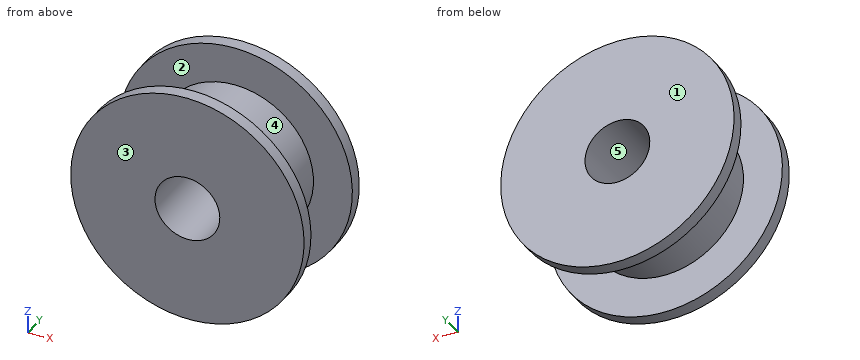
from build123d import *

# Parameters (mm, degrees)
SKETCH1_R           = 9
BOSS_EXTRUDE1_DEPTH = 8
SKETCH3_R           = 2.5
CUT_EXTRUDE1_DEPTH  = 16.033296378
SKETCH2_W           = 3
SKETCH2_H           = 6


with BuildPart() as part:
    # Sketch1 → Boss-Extrude1 (new body)
    with BuildSketch(Plane(origin=(0, 0, 0), x_dir=(1, 0, 0), z_dir=(0, 1, 0))):
        with Locations(Location((0, 0, 0), (0, 0, 270))):
            Circle(SKETCH1_R)
    extrude(amount=BOSS_EXTRUDE1_DEPTH)

    # Sketch3 → Cut-Extrude1 (cut, through all)
    with BuildSketch(Plane(origin=(0, 8, 0), x_dir=(1, 0, 0), z_dir=(0, 1, 0))):
        with Locations(Location((0, 0, 0), (0, 0, 270))):
            Circle(SKETCH3_R)
    extrude(amount=-CUT_EXTRUDE1_DEPTH, mode=Mode.SUBTRACT)

    # Sketch2 → Cut-Revolve1 (revolve, cut)
    with BuildSketch(Plane(origin=(0, 0, 0), x_dir=(0, 0, -1), z_dir=(1, 0, 0)), mode=Mode.PRIVATE) as cut_revolve1_sk:
        with Locations((-7.5, 4)):
            Rectangle(SKETCH2_W, SKETCH2_H)
    revolve(cut_revolve1_sk.sketch.rotate(Axis((0, 0, 0), (0, 1, 0)), 180), axis=Axis((0, 0, 0), (0, 1, 0)), mode=Mode.SUBTRACT)


solid = part.part
Verification items for the finished model (mm, model axes). Face numbers are marked on the shaded views. A direction names the side the tool comes from. Give positions to 0.01 mm unless a question says otherwise; leave off trailing zeros. Write each loop counter-clockwise with the first axis right and the second up, starting at its lowest first coordinate (ties: lowest second). Pieces come first, ordered by that corner, then holes.
(1) Gauge pin test, flat ends, axial feed: pin 1 (4 mm diameter, centred on x = 0.5, z = 2, fed in from +Y); pin 2 (3 mm diameter, centred on x = 2.5, y = 1, fed in from -Z). Record the tip position at first contact, or that the pin passes through.
(2) Cross-section at D-D (z = 8). Enter the section's corners in (x, y).
(3) Cross-section at C-C (y = 5.25). Enter the section's corners in (x, z), plus the area to 3 significant figures.
(4) Access from +Z, -Z, +X, -X, +Y, -Y to the whole of each face (thin tool, end or side, straight path). Record for the marked faces 1 and 2.
(5) Cross-section at A-A (z = 0). Enter the section's corners in (x, y), plus the area to 3 significant figures.
(6) Cross-section at B-B (x = 0). Enter the section's corners in (y, z), plus the area to 3 significant figures.
(7) Mould release check, pull along Z, two halves, no side actions. Record for the marked faces 3, 4 and 5: +Z half, -Z half, draft (parallel to the pull), parting line (faces both ways), or undercut.
(8) Material ranges on line 1 (Y direction, x = 8, z = -1.25); line 2 (X direction, y = 3.5, z = 0); line 3 (Z direction, x = 1, y = 5), recorded low to high.
Worked out:
1. pin 1: stops at y = 8
1. pin 2: stops at z = -8.94
2. outline: (-4.12, 0) - (4.12, 0) - (4.12, 1) - (-4.12, 1) - close; (-4.12, 7) - (4.12, 7) - (4.12, 8) - (-4.12, 8) - close
3. outline: circle Ø12 at (0, 0); hole circle Ø5 at (0, 0)
3. area: 93.5 mm2
4. face 1: +Z, -Z, +X, -X, +Y
4. face 2: none
5. outline: (-9, 0) - (-2.5, 0) - (-2.5, 8) - (-9, 8) - (-9, 7) - (-6, 7) - (-6, 1) - (-9, 1) - close; (2.5, 0) - (9, 0) - (9, 1) - (6, 1) - (6, 7) - (9, 7) - (9, 8) - (2.5, 8) - close
5. area: 68.0 mm2
6. outline: (0, -9) - (1, -9) - (1, -6) - (7, -6) - (7, -9) - (8, -9) - (8, -2.5) - (0, -2.5) - close; (0, 2.5) - (8, 2.5) - (8, 9) - (7, 9) - (7, 6) - (1, 6) - (1, 9) - (0, 9) - close
6. area: 68.0 mm2
7. face 3: draft
7. face 4: parting line
7. face 5: undercut
8. line 1: y = 0 to 1, 7 to 8
8. line 2: x = -6 to -2.5, 2.5 to 6
8. line 3: z = -5.92 to -2.29, 2.29 to 5.92
